Geometry: see drawing. Coordinates: mm, zero at the bounding-box minimum. Coordinates: 2 decimals unless noted, no trailing zeros. Write each loop counter-clockwise with the first axis right and the second up, starting at its lowest first coordinate (ties: lowest second). Pieces come first, ordered by that corner, then holes. Notation, with made-up numbers: M 7.25,19 L 14.25,19 A23 ccw 14.25,31 Z; hole C 68.5,-36 d8. An arc over 180 degrees is marked long. One line per item, written item: value. Start each with the question number.
Item 1: Cut plane B-B, the plane x = 2.5. Output: boundary loops of the cut face in (y, z), then the cut area to 3 significant figures.
Item 2: Ray query, L1, parallel to Y at x = 2.5, z = 2.2; L2, parallel to Y at x = 1.95, z = 2.6; L3, parallel to X at y = 1, z = 3.3. Return the intervals inside material, ascending. Write a range as from..to.
Item 3: Mould query, pull axis Y, two halves, no side actions, for the marked faces 1, 2 and 3. Classes: released by +Y, released by -Y, zero draft, split by the parting line, or undercut.
Item 4: Cut plane C-C, the plane z = 2.3. Output: boundary loops of the cut face in (x, y), then the cut area to 3 significant figures.
Item 5: Pin query (flat end, axial travel): P1, Ø2.5, axis at x = 2.5, y = 12.5, coming from the +Z side; P2, Ø2, axis at y = 3, z = 3, coming from the -X side. Return the tip coordinate at first contact, or that it passes through.
Item 6: Cut plane A-A, the plane y = 12.5. Output: boundary loops of the cut face in (x, z), then the cut area to 3 significant figures.
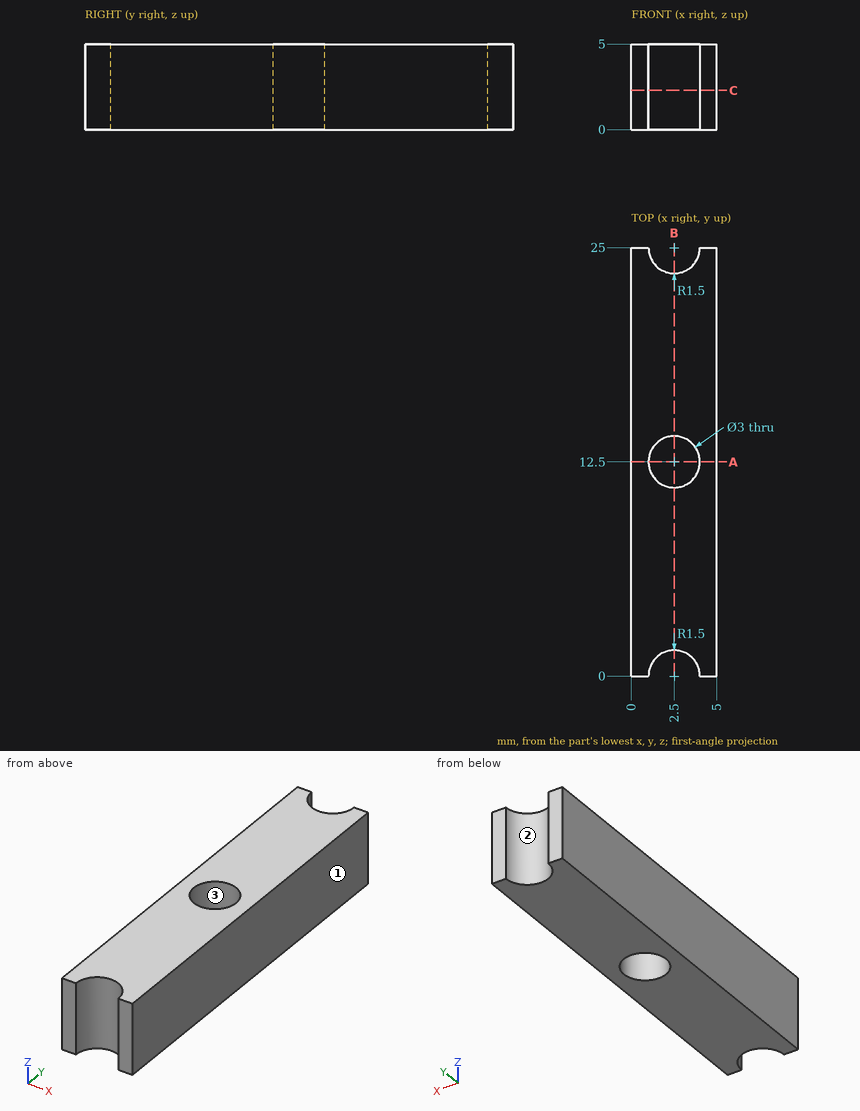
From the geometry:
1. outline: M 1.5,0 L 11,0 L 11,5 L 1.5,5 Z; M 14,0 L 23.5,0 L 23.5,5 L 14,5 Z
1. area: 95.0 mm²
2. L1: y = 1.5..11, 14..23.5
2. L2: y = 1.4..11.1, 13.9..23.6
2. L3: x = 0..1.38, 3.62..5
3. face 1: zero draft
3. face 2: released by +Y
3. face 3: undercut
4. outline: M 0,0 L 1,0 A1.5 cw 4,0 L 5,0 L 5,25 L 4,25 A1.5 cw 1,25 L 0,25 Z; hole C 2.5,12.5 d3
4. area: 111 mm²
5. P1: passes through
5. P2: stops at x = 0
6. outline: M 0,0 L 1,0 L 1,5 L 0,5 Z; M 4,0 L 5,0 L 5,5 L 4,5 Z
6. area: 10.0 mm²
